Read the model definition and answer for the solid it produces. Units are mm, in the model's axes. A direction names the side the tool comes from. Round coordinates to 2 decimals unless told otherwise and drop trailing zeros.
from build123d import *

# Parameters (mm, degrees)
CROQUIS2_R              = 2
SALIENTE_EXTRUIR1_DEPTH = 5
MATRIZC6_COUNT          = 10


with BuildPart() as part:
    # Croquis2 → Saliente-Extruir1 (new body)
    with BuildSketch(Plane.XY):
        with BuildLine():
            Line((-0.306026412, 5.044473868), (0, 5.87307888))
            add(Edge.make_bspline(
                [(0, 5.87307888), (0.02679779, 6.141175495), (0.274936867, 6.703868053), (0.663188036, 7.188067029), (0.910477928, 7.4337912), (0.9201705, 7.443338381)],
                knots=[0, 0, 0, 0, 0.049397205, 0.111126444, 0.113633344, 0.113633344, 0.113633344, 0.113633344], degree=3))
            ThreePointArc((0.9201705, 7.443338381), (1.246914914, 7.395620542), (1.571242221, 7.333566519))
            add(Edge.make_bspline(
                [(1.976598848, 5.530471275), (2.031114418, 5.617400913), (2.087789883, 5.844644836), (2.081168958, 6.255490925), (1.933755754, 6.776716333), (1.720527283, 7.138546833), (1.576032848, 7.327357984), (1.571242221, 7.333566519)],
                knots=[0, 0, 0, 0, 0.049397205, 0.111126444, 0.197545762, 0.30865546, 0.312445362, 0.312445362, 0.312445362, 0.312445362], degree=3))
            Line((1.976598848, 5.530471275), (1.814118887, 4.552477655))
            ThreePointArc((1.814118887, 4.552477655), (1.827796208, 4.471943871), (1.888292818, 4.417053803))
            ThreePointArc((1.888292818, 4.417053803), (-0.82041007, -4.733174556), (-0.291568658, 4.794893302))
            ThreePointArc((-0.291568658, 4.794893302), (-0.174364868, 4.926891746), (-0.306026412, 5.044473868))
        make_face()
        Circle(CROQUIS2_R, mode=Mode.SUBTRACT)
    saliente_extruir1 = extrude(amount=SALIENTE_EXTRUIR1_DEPTH)

    # MatrizC6: Saliente-Extruir1 ×10 about axis
    matrizc6_axis = Axis((0, 0, 5), (0, 0, -1))
    for i in range(1, MATRIZC6_COUNT):
        add(saliente_extruir1.rotate(matrizc6_axis, i * 360 / MATRIZC6_COUNT))


solid = part.part
Q1. Which of the six approach directions +Z, -Z, +X, -X, +Y, -Y give full straight-line access (tool end or side, diameter ignored) to faces 1 (the flat face through (-0.155, 5.453, 2.465)), 2 (the flat face through (4.215, -3.364, 2.465)), 3 (the flat face through (-1.896, -5.048, 2.465))?
Verdict:
face 1: +Z, -Z, +Y
face 2: +Z, -Z, -Y
face 3: +Z, -Z
Q2. Straight lines are drawn through the part: probe 1 along X at (y, z) = (0.75, 1.85); probe 2 along Y at (x, z) = (5.25, 3.35); probe 3 along X at (y, z) = (0, 1.3). For each, find the intervals that lie inside material, in ascending order.
Verdict:
probe 1: x = -4.74 to -1.85, 1.85 to 7.45
probe 2: y = -3.88 to -1.55, -0.26 to 1.83, 3.69 to 5.36
probe 3: x = -6.64 to -2, 2 to 6.64
Q3. Determine the mould class of faces 4 (the flat face through (-0.3, -2.2, 5)), 5 (the flat face through (-1.433, 5.199, 2.465)), 6 (the flat face through (-4.215, 3.364, 2.465)) for opening direction X: pulls with the +X half, pulls with the -X half, needs draft (parallel to the pull), parting line crosses it, or undercut.
Verdict:
face 4: needs draft
face 5: undercut
face 6: undercut
Q4. Flat-ended cylindrical pins translate along their axes: pin 1 Ø2 at (y, z) = (3.5, 4.5) entering from +X; pin 2 Ø1.5 at (x, z) = (-3, 3.5) entering from +Y; pin 3 Ø1 at (y, z) = (4, 2.5) entering from -X. Find the tip coordinate at first contact, or state that the pin passes through.
Verdict:
pin 1: stops at x = 5.55
pin 2: stops at y = 6.86
pin 3: stops at x = -6.63
